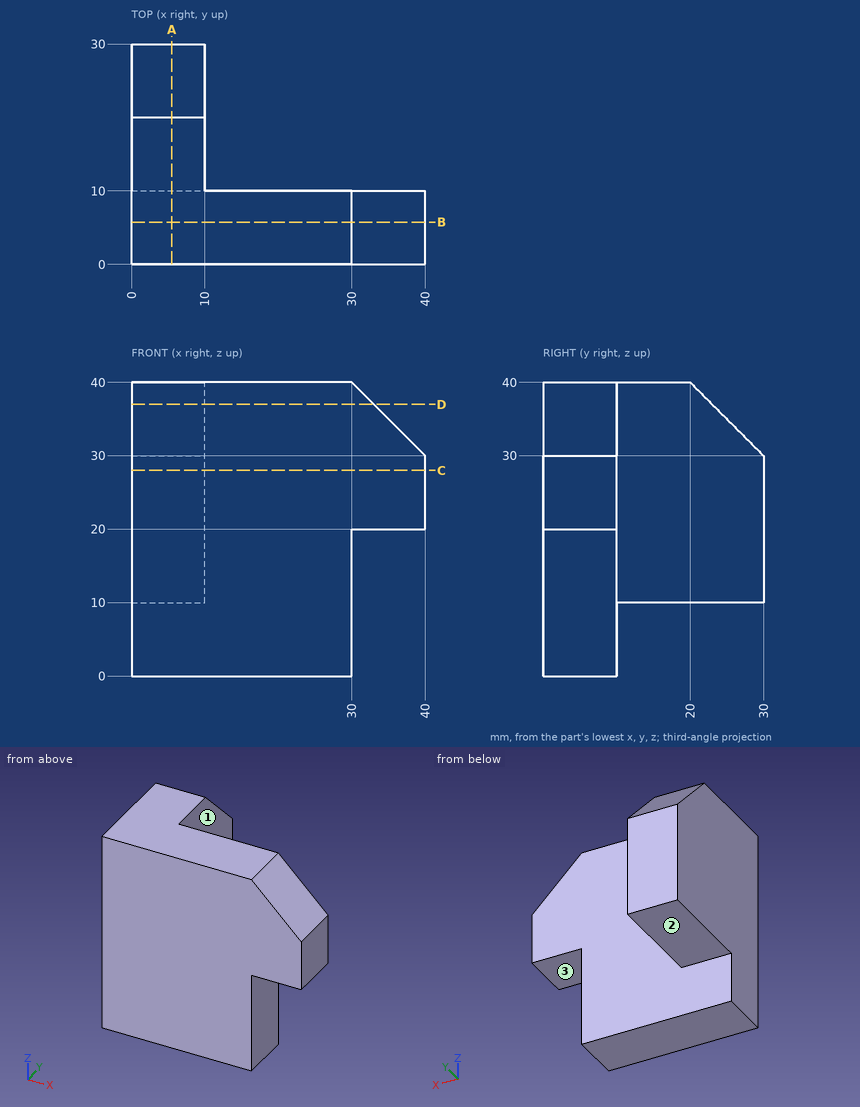
Geometry: see drawing. Coordinates: mm, zero at the bounding-box minimum. A direction names the side the tool comes from. Coordinates: 2 decimals unless noted, no trailing zeros. Write each loop counter-clockwise with the first axis right and the second up, starting at its lowest first coordinate (ties: lowest second). Pieces come first, ordered by that corner, then holes. Notation, with made-up numbers: (20.5, -31) - (24.5, -31) arc R20 ccw to (24.5, -12) - close; hole circle Ø4 at (16, 49). An arc over 180 degrees is marked (long way). Put each result on its own line as item: value. Start each with the question number.
1) Reachability of the marked faces 1, 2 and 3 from +Z, -Z, +X, -X, +Y, -Y: full face, straight path, thin tool, end or side. Return the list, or none.
2) Cut plane C-C (z = 28). Return the cut outline in (x, y), plus the area to 3 significant figures.
3) Cut plane A-A (x = 5.5). Return the cut outline in (y, z), plus the area to 3 significant figures.
4) Cut plane B-B (y = 5.75). Return the cut outline in (x, z).
5) Contact query for flat-ended pins moving along their axis: pin 1 (1.5 mm diameter, centred on y = 12.5, z = 14.5, fed in from +X); pin 2 (6 mm diameter, centred on x = 33.5, z = 20, fed in from +Y); pin 3 (11 mm diameter, centred on x = 34.5, y = 4.5, fed in from -Z); pin 4 (5 mm diameter, centred on x = 34, y = 4, fed in from -Z). Output: stop coordinate, or through.
6) Cut plane D-D (z = 37). Return the cut outline in (x, y), plus the area to 3 significant figures.
7) Ray query, L1, parallel to X at y = 18.25, z = 30; L2, parallel to Y at x = 8.5, z = 37. Return the intervals inside material, ascending.
Resolved:
1. face 1: +Z, -Z, +X, +Y
1. face 2: -Z, +X, -X, +Y
1. face 3: -Z, +X, +Y, -Y
2. outline: (0, 0) - (40, 0) - (40, 10) - (10, 10) - (10, 30) - (0, 30) - close
2. area: 600 mm2
3. outline: (0, 0) - (10, 0) - (10, 10) - (30, 10) - (30, 30) - (20, 40) - (0, 40) - close
3. area: 950 mm2
4. outline: (0, 0) - (30, 0) - (30, 20) - (40, 20) - (40, 30) - (30, 40) - (0, 40) - close
5. pin 1: stops at x = 10
5. pin 2: stops at y = 10
5. pin 3: stops at z = 0
5. pin 4: stops at z = 20
6. outline: (0, 0) - (33, 0) - (33, 10) - (10, 10) - (10, 23) - (0, 23) - close
6. area: 460 mm2
7. L1: x = 0 to 10
7. L2: y = 0 to 23
